Check sheet for the drawn part. Datum: minimum x, y, z corner. Units: mm. A direction names the side the tool comes from. Give positions to 0.01 mm unless a question says otherwise; leave off trailing zeros. Write each loop counter-clockwise with the first axis right and the second up, starting at its lowest first coordinate (ties: lowest second). Pieces come first, ordered by that corner, then holes.
(1) Tool access check on the marked faces 5 and 6. Record the directions out of +Z, -Z, +X, -X, +Y, -Y that give a thin tool (end or side, any length) a straight path to the whole face; none if there is none.
(2) Mould release check, pull along Z, two halves, no side actions. Record for the marked faces 1, 2, 3 and 4: +Z half, -Z half, draft (parallel to the pull), parting line (faces both ways), or undercut.
(3) Depth check by flat-ended pin: P1, Ø1.5, axis at x = 11.5, y = 2, coming from the +Z side. Enter the tip coordinate at first touch or a pass-through.
(4) Cross-section at C-C (y = 6.25). Record the boundary of the cut face in (x, z).
(5) Cross-section at B-B (z = 9.25). Record the boundary of the cut face in (x, y).
(6) Thickness scan on line 1 along Z through (x, y) = (25, 2.5); line 2 along X through (y, z) = (3.5, 12.5); line 3 along X through (y, z) = (5, 10.5). Record the ranges inside material, lowest first.
(7) Cross-section at D-D (z = 5.75). Record the boundary of the cut face in (x, y).
(8) Cross-section at A-A (x = 25). Record the boundary of the cut face in (y, z), and give its area (3 significant figures).
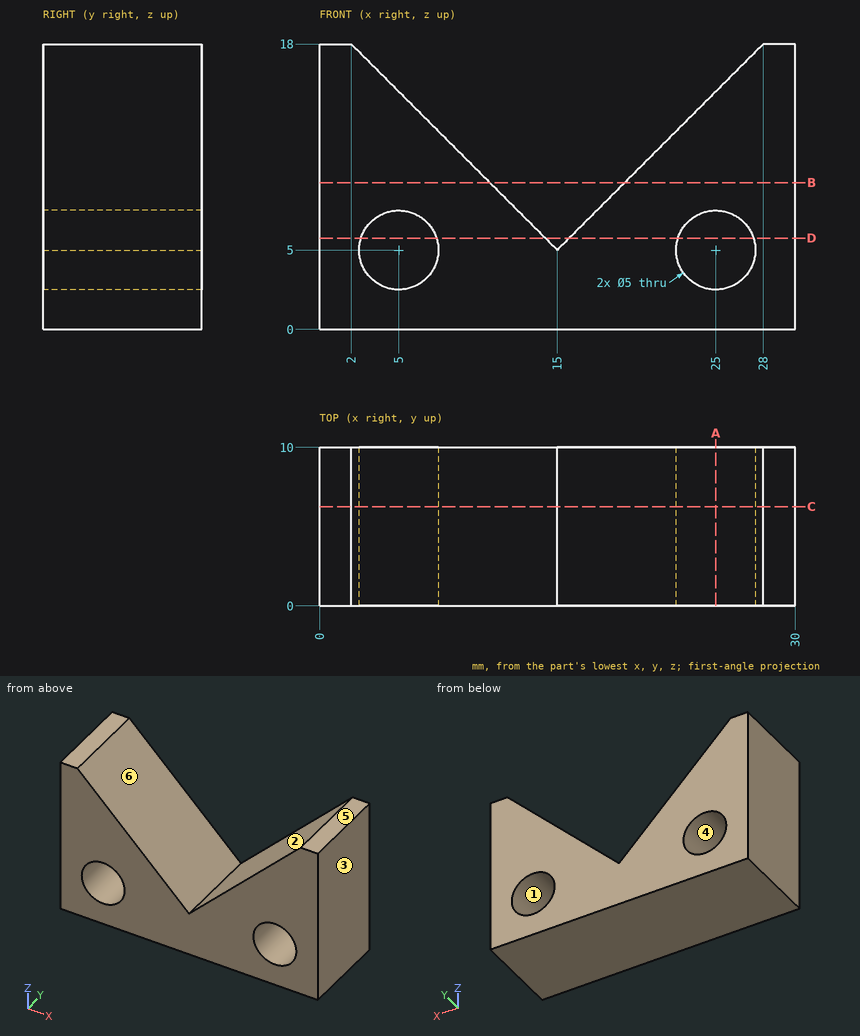
Reply:
1. face 5: +Z, +X, -X, +Y, -Y
1. face 6: +Z, +Y, -Y
2. face 1: undercut
2. face 2: +Z half
2. face 3: draft
2. face 4: undercut
3. P1: stops at z = 9.25
4. outline: (0, 0) - (30, 0) - (30, 18) - (28, 18) - (15, 5) - (2, 18) - (0, 18) - close; hole circle Ø5 at (5, 5); hole circle Ø5 at (25, 5)
5. outline: (0, 0) - (10.75, 0) - (10.75, 10) - (0, 10) - close; (19.25, 0) - (30, 0) - (30, 10) - (19.25, 10) - close
6. line 1: z = 0 to 2.5, 7.5 to 15
6. line 2: x = 0 to 7.5, 22.5 to 30
6. line 3: x = 0 to 9.5, 20.5 to 30
7. outline: (0, 0) - (2.62, 0) - (2.62, 10) - (0, 10) - close; (7.38, 0) - (14.25, 0) - (14.25, 10) - (7.38, 10) - close; (15.75, 0) - (22.62, 0) - (22.62, 10) - (15.75, 10) - close; (27.38, 0) - (30, 0) - (30, 10) - (27.38, 10) - close
8. outline: (0, 0) - (10, 0) - (10, 2.5) - (0, 2.5) - close; (0, 7.5) - (10, 7.5) - (10, 15) - (0, 15) - close
8. area: 100 mm2
